```python
from build123d import *

# Parameters (mm, degrees)
EXTRUDE_1_DEPTH = 2


with BuildPart() as part:
    # 草图1 → 凸台-拉伸1 (new body)
    with BuildSketch(Plane(origin=(0, 0, 0), x_dir=(1, 0, 0), z_dir=(0, 1, 0))):
        with BuildLine():
            Line((0, 0), (125.7, 0))
            Line((125.7, 0), (125.7, -77.7))
            Line((125.7, -77.7), (79.265, -77.7))
            Line((79.265, -77.7), (72.35, -63.178332735))
            ThreePointArc((72.35, -63.178332735), (62.85, -57.18), (53.35, -63.178332735))
            Line((53.35, -63.178332735), (46.435, -77.7))
            Line((46.435, -77.7), (0, -77.7))
            Line((0, -77.7), (0, 0))
        make_face()
        with BuildLine():
            ThreePointArc((9.647969095, -36.353809997), (20.835, -19.234524604), (41.254251498, -18.105914344))
            ThreePointArc((41.254251498, -18.105914344), (42.235, -21.399588114), (45.577779407, -20.602104347))
            ThreePointArc((45.577779407, -20.602104347), (54.81, -38.85), (45.577779407, -57.097895653))
            ThreePointArc((45.577779407, -57.097895653), (42.235, -56.300411886), (41.254251498, -59.594085656))
            ThreePointArc((41.254251498, -59.594085656), (20.835, -58.465475396), (9.647969095, -41.346190003))
            ThreePointArc((9.647969095, -41.346190003), (12.01, -38.85), (9.647969095, -36.353809997))
        make_face(mode=Mode.SUBTRACT)
        with BuildLine():
            ThreePointArc((80.122220593, -57.097895653), (83.465, -56.300411886), (84.445748502, -59.594085656))
            ThreePointArc((84.445748502, -59.594085656), (104.865, -58.465475396), (116.052030905, -41.346190003))
            ThreePointArc((116.052030905, -41.346190003), (113.69, -38.85), (116.052030905, -36.353809997))
            ThreePointArc((116.052030905, -36.353809997), (104.865, -19.234524604), (84.445748502, -18.105914344))
            ThreePointArc((84.445748502, -18.105914344), (83.465, -21.399588114), (80.122220593, -20.602104347))
            ThreePointArc((80.122220593, -20.602104347), (70.89, -38.85), (80.122220593, -57.097895653))
        make_face(mode=Mode.SUBTRACT)
    extrude(amount=EXTRUDE_1_DEPTH)


solid = part.part
```
The listing builds one solid part. Answer for the finished solid, in the listing's coordinates (mm). A direction names the side the tool comes from. Coordinates: 2 decimals unless noted, no trailing zeros. Loops run counter-clockwise (first coordinate to the right, second up) from the corner with the lowest first, then second, coordinate; pieces in that order, holes last. Notation, with made-up numbers: (86.25, 33) -> (93.25, 33) arc R19 cw to (93.25, 49) -> close; hole circle Ø2 at (31.25, -23.5). An arc over 180 degrees is marked (long way). Return JSON: item names as keys, results as strings. Group by question number.
(1) Find the intervals of material crossed by probe 1 along X at (y, z) = (0.6, 39); probe 2 along X at (y, z) = (1.05, 21); probe 3 along X at (y, z) = (0.85, 42), in increasing order. Write a range as from..to.
(2) A cutting plane is placed at C-C on x = 48.5. Write down the section's boundary in (y, z), and give its area (3 significant figures).
(3) A cutting plane is placed at B-B on y = 0.85. Write down the section's boundary in (x, z) (3 decimals).
(4) Given pin 1 Ø8 at (x, z) = (77, 25) entering from +Y, flat-ended and moving along its own axis, determine where the tip first touches the part or whether it passes through.
(5) Determine the mould class of faces 1 (the flat face through (64, 2, 38)), 2 (the flat face through (49.94, 0.99, 70.34)), 3 (the cylindrical face through (54.81, 0.99, 38.55)) for opening direction Z: released by +Z, released by -Z, zero draft, split by the parting line, or undercut.
(6) A cutting plane is placed at D-D on z = 70.5. Write down the section's boundary in (x, y).
(7) A cutting plane is placed at A-A on z = 38.85. Write down the section's boundary in (x, y), and give its area (3 significant figures).
(8) Which of the six approach directions +Z, -Z, +X, -X, +Y, -Y give full straight-line access (tool end or side, diameter ignored) to faces 4 (the flat face through (64, 0, 38)), 5 (the flat face through (75.856, 0.986, 70.541)), 6 (the cylindrical face through (21.09, 0.99, 58.61))?
The answers:
{
 "1": {"probe 1": "x = 0..12.01, 54.81..70.89, 113.69..125.7", "probe 2": "x = 0..18.22, 41.71..45.26, 46.1..79.6, 80.44..83.99, 107.48..125.7", "probe 3": "x = 0..9.73, 54.59..71.11, 115.97..125.7"},
 "2": {"outline": "(0, 0) -> (2, 0) -> (2, 23.16) -> (0, 23.16) -> close; (0, 54.54) -> (2, 54.54) -> (2, 73.36) -> (0, 73.36) -> close", "area": "84.0 mm^2"},
 "3": {"outline": "(0, 0) -> (125.7, 0) -> (125.7, 77.7) -> (79.265, 77.7) -> (72.35, 63.178) arc R10.522 cw to (53.35, 63.178) -> (46.435, 77.7) -> (0, 77.7) -> close; hole (9.648, 36.354) arc R22.65 ccw to (41.254, 18.106) arc R2.5 cw to (45.578, 20.602) arc R22.65 ccw to (45.578, 57.098) arc R2.5 cw to (41.254, 59.594) arc R22.65 ccw to (9.648, 41.346) arc R2.5 cw to start; hole (80.122, 20.602) arc R2.5 cw to (84.446, 18.106) arc R22.65 ccw to (116.052, 36.354) arc R2.5 cw to (116.052, 41.346) arc R22.65 ccw to (84.446, 59.594) arc R2.5 cw to (80.122, 57.098) arc R22.65 ccw to start"},
 "4": {"pin 1": "stops at y = 2"},
 "5": {"face 1": "zero draft", "face 2": "released by +Z", "face 3": "undercut"},
 "6": {"outline": "(0, 0) -> (49.86, 0) -> (49.86, 2) -> (0, 2) -> close; (75.84, 0) -> (125.7, 0) -> (125.7, 2) -> (75.84, 2) -> close"},
 "7": {"outline": "(0, 0) -> (12.01, 0) -> (12.01, 2) -> (0, 2) -> close; (54.81, 0) -> (70.89, 0) -> (70.89, 2) -> (54.81, 2) -> close; (113.69, 0) -> (125.7, 0) -> (125.7, 2) -> (113.69, 2) -> close", "area": "80.2 mm^2"},
 "8": {"face 4": "+Z, -Z, +X, -X, -Y", "face 5": "+Z, +Y, -Y", "face 6": "+Y, -Y"}
}
